Part print with two shaded views. Sizes in mm from the minimum x, y, z corner. A direction names the side the tool comes from. Give positions to 0.01 mm unless a question says otherwise; leave off trailing zeros. Loops run counter-clockwise (first coordinate to the right, second up) from the corner with the lowest first, then second, coordinate; pieces in that order, holes last. Notation, with made-up numbers: M 32.25,88 L 73.25,88 A7 cw 73.25,92 Z; hole C 8,49 d1. An arc over 180 degrees is marked long. Answer as a JSON object with one key per item and string values. Group by question number.
1. Slice it at A-A (z = 7.5). List the corners of the cut face in (x, y), then the cut area to 3 significant figures.
2. Slice it at C-C (y = 32). List the corners of the cut face in (x, z).
3. 3-axis set-ups, long thin cutter, end or side, ignore diameter. For the marked faces 1 and 2: which of +Z, -Z, +X, -X, +Y, -Y reach the whole face in a straight line?
4. Drill centre lines: line 1 along Y through (x, z) = (56, 7); line 2 along Y through (x, z) = (25, 5); line 3 along X through (y, z) = (15.5, 10). Where is each one in solid material? Low to high. Write a range as [from, to].
5. Drop flat-ended pins along their axis: pin 1 Ø15.5 at (x, y) = (53, 27.5) entering from +Z; pin 2 Ø2 at (x, y) = (35, 10.5) entering from -Z; pin 3 Ø1.3 at (x, z) = (64, 2.5) entering from -Y. Give the stop position or say it passes through.
6. Slice it at D-D (y = 44). List the corners of the cut face in (x, z), then the cut area to 3 significant figures.
7. Mould opens along X. For the marked faces 3, 4 and 5 say: released by +X, released by -X, zero draft, split by the parting line, or undercut.
8. Slice it at B-B (x = 56). List the corners of the cut face in (y, z), then the cut area to 3 significant figures.
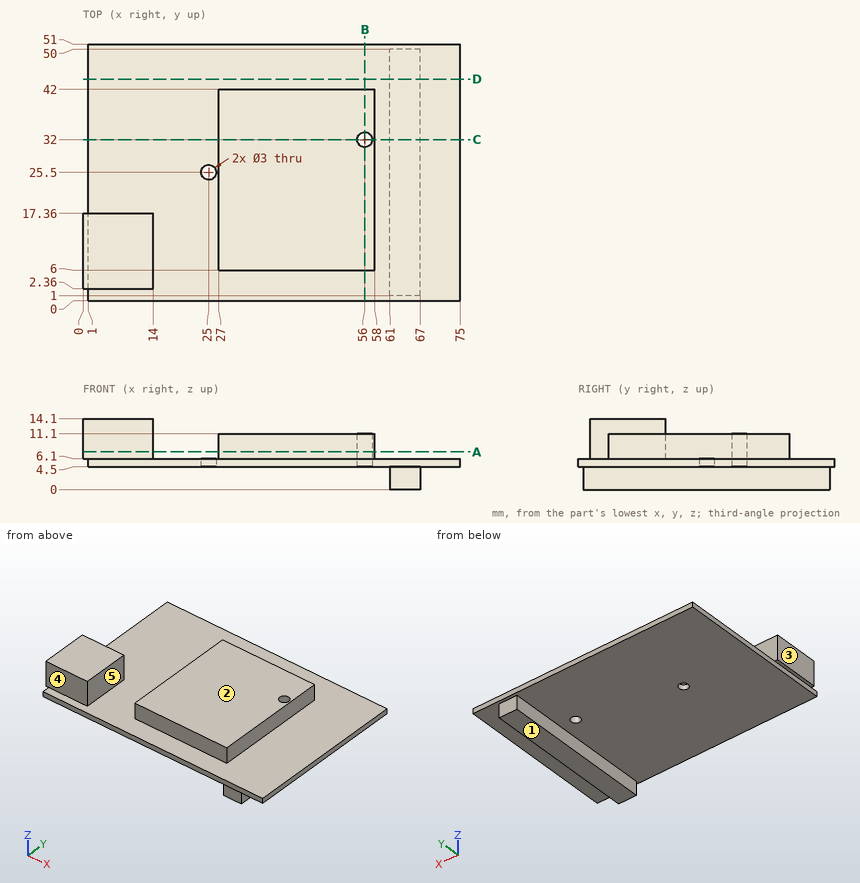
Established:
{
 "1": {"outline": "M 0,2.36 L 14,2.36 L 14,17.36 L 0,17.36 Z; M 27,6 L 58,6 L 58,42 L 27,42 Z; hole C 56,32 d3", "area": "1,320 mm^2"},
 "2": {"outline": "M 1,4.5 L 54.5,4.5 L 54.5,11.1 L 27,11.1 L 27,6.1 L 1,6.1 Z; M 57.5,4.5 L 61,4.5 L 61,0 L 67,0 L 67,4.5 L 75,4.5 L 75,6.1 L 58,6.1 L 58,11.1 L 57.5,11.1 Z"},
 "3": {"face 1": "-Z, +X, -X, +Y, -Y", "face 2": "+Z, +X, +Y, -Y"},
 "4": {"line 1": "y = [6, 30.5], [33.5, 42]", "line 2": "y = [0, 24], [27, 51]", "line 3": "x = [0, 14], [27, 58]"},
 "5": {"pin 1": "stops at z = 11.1", "pin 2": "stops at z = 4.5", "pin 3": "stops at y = 1"},
 "6": {"outline": "M 1,4.5 L 61,4.5 L 61,0 L 67,0 L 67,4.5 L 75,4.5 L 75,6.1 L 1,6.1 Z", "area": "145 mm^2"},
 "7": {"face 3": "released by -X", "face 4": "zero draft", "face 5": "undercut"},
 "8": {"outline": "M 0,4.5 L 30.5,4.5 L 30.5,11.1 L 6,11.1 L 6,6.1 L 0,6.1 Z; M 33.5,4.5 L 51,4.5 L 51,6.1 L 42,6.1 L 42,11.1 L 33.5,11.1 Z", "area": "242 mm^2"}
}
